Can you work these out from the model? Positions are in its coordinate system, mm. Give positions to 0.01 mm unless a question says otherwise; leave off trailing zeros. Loops run counter-clockwise (first coordinate to the right, second up) from the corner with the lowest first, then second, coordinate; pieces in that order, holes last. Notation, with made-up numbers: (89.25, 73.25) - (129.25, 73.25) arc R21 ccw to (129.25, 92.25) - close; hole circle Ø10 at (87.5, 61.5). An arc over 180 degrees is marked (long way). Answer in a Markdown table with one row per item.
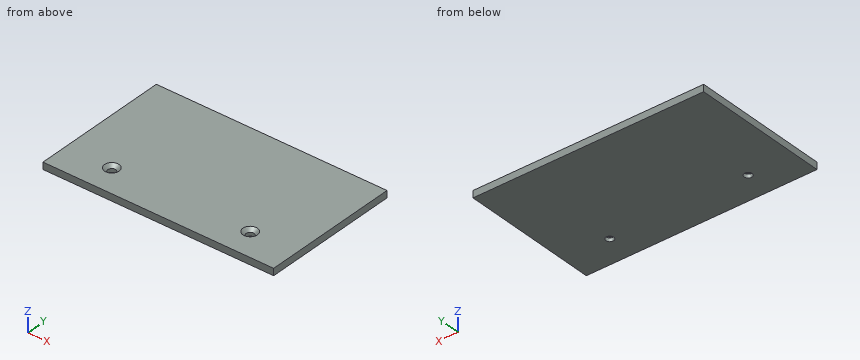
from build123d import *

# Parameters (mm, degrees)
SKETCH1_W                                    = 100
SKETCH1_H                                    = 60
BOSS_EXTRUDE1_DEPTH                          = 1.5
CSK_FOR_M3_COUNTERSUNK_FLAT_HEAD_SCR_2_COUNT = 2
CSK_FOR_M3_COUNTERSUNK_FLAT_HEAD_SCR_2_PITCH = 60


with BuildPart() as part:
    # Sketch1 → Boss-Extrude1 (new, symmetric)
    with BuildSketch(Plane.XY):
        Rectangle(SKETCH1_W, SKETCH1_H)
    extrude(amount=BOSS_EXTRUDE1_DEPTH, both=True)

    # Sketch3 → CSK for M3 Countersunk Flat Head Screw1 (revolve, cut)
    with BuildSketch(Plane(origin=(-30, -18, 1.5), x_dir=(0, -1, 0), z_dir=(1, 0, 0))):
        Polygon((0, 0), (0, 3), (1.7, 3), (1.7, 1.45), (3.15, 0), align=None)
    csk_for_m3_countersunk_flat_head_screw1 = revolve(axis=Axis((-30, -18, 7.85), (0, 0, -1)), mode=Mode.SUBTRACT)

    # CSK for M3 Countersunk Flat Head Scr 2: CSK for M3 Countersunk Flat Head Screw1 ×2
    with Locations(*[(i * CSK_FOR_M3_COUNTERSUNK_FLAT_HEAD_SCR_2_PITCH, 0, 0) for i in range(1, CSK_FOR_M3_COUNTERSUNK_FLAT_HEAD_SCR_2_COUNT)]):
        add(csk_for_m3_countersunk_flat_head_screw1, mode=Mode.SUBTRACT)


solid = part.part
Q1. If I drill on line 1 (X direction, y = -18, z = -1.05); line 2 (Y direction, x = -30, z = -0.45); line 3 (Y direction, x = -30, z = 0.75), over which ranges is the centre line in solid material (lowest first)? Write a range as [from, to].
Checked values:
| item | result |
|---|---|
| line 1 | x = [-50, -31.7], [-28.3, 28.3], [31.7, 50] |
| line 2 | y = [-30, -19.7], [-16.3, 30] |
| line 3 | y = [-30, -20.4], [-15.6, 30] |
Q2. Imagine slicing it at A-A, the plane x = 30. Write out the boundary of the cut face in (y, z), and give its area (3 significant figures).
Checked values:
| item | result |
|---|---|
| outline | (-30, -1.5) - (-19.7, -1.5) - (-19.7, 0.05) - (-21.15, 1.5) - (-30, 1.5) - close; (-16.3, -1.5) - (30, -1.5) - (30, 1.5) - (-14.85, 1.5) - (-16.3, 0.05) - close |
| area | 168 mm² |
Q3. Imagine slicing it at B-B, the plane y = -18. Write out the boundary of the cut face in (x, z).
Checked values:
| item | result |
|---|---|
| outline | (-50, -1.5) - (-31.7, -1.5) - (-31.7, 0.05) - (-33.15, 1.5) - (-50, 1.5) - close; (-28.3, -1.5) - (28.3, -1.5) - (28.3, 0.05) - (26.85, 1.5) - (-26.85, 1.5) - (-28.3, 0.05) - close; (31.7, -1.5) - (50, -1.5) - (50, 1.5) - (33.15, 1.5) - (31.7, 0.05) - close |
Q4. For pin 1 (4.5 mm diameter, centred on x = 30, y = -18, fed in from +Z), with a flat end and sliding along its axis, tell me the tip position at first contact or that it passes through.
Checked values:
| item | result |
|---|---|
| pin 1 | stops at z = 0.6 |
